For this review, take the finished solid that the model builds, in its own axes (mm). Face numbers are marked on the shaded views. A direction names the side the tool comes from. Coordinates: 2 decimals unless noted, no trailing zeros. Order: outer loops, then holes, each group sorted by start corner. A loop starts at its lowest first (then second) coordinate and runs counter-clockwise, first axis right, second up. Notation, with made-up numbers: M -18.5,86.5 L -5.5,86.5 A14 ccw -5.5,104.5 Z; hole C -18.75,46 d1. An arc over 180 degrees is marked long. Use one line per item in the form item = value. Start each with the question number.
```python
from build123d import *

# Parameters (mm, degrees)
HEX_CUT_DEPTH = 3.048
CHAMFER2_SIZE = 0.381


with BuildPart() as part:
    # Base Sketch → Base (revolve)
    with BuildSketch(Plane.XY, mode=Mode.PRIVATE) as base_sk:
        Polygon((0, 0), (25.4, 0), (25.4, 4.7625), (19.05, 4.7625), (19.05, 3.175), (0, 3.175), align=None)
    revolve(base_sk.sketch.rotate(Axis((0, 0, 0), (1, 0, 0)), 90), axis=Axis((0, 0, 0), (1, 0, 0)))

    # Hex Sketch → Hex Cut (cut)
    with BuildSketch(Plane(origin=(25.4, 0, 0), x_dir=(0, 0, -1), z_dir=(1, 0, 0))):
        Polygon((-1.374815329, 2.38125), (-2.749630657, 0), (-1.374815329, -2.38125), (1.374815329, -2.38125), (2.749630657, 0), (1.374815329, 2.38125), align=None)
    extrude(amount=-HEX_CUT_DEPTH, mode=Mode.SUBTRACT)

    # Chamfer2
    chamfer2_edges = [part.edges().sort_by_distance(p)[0] for p in [
        (0, 0, -3.175),
        (19.05, 0, -4.7625),
        (25.4, 0, -4.7625),
    ]]
    chamfer(chamfer2_edges, length=CHAMFER2_SIZE)


solid = part.part
```
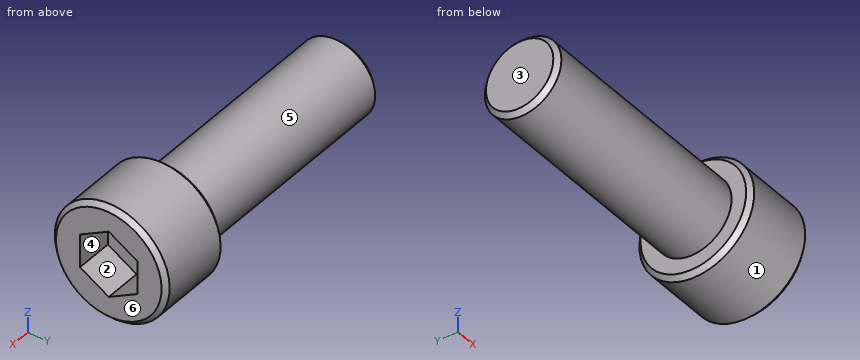
1. For pin 1 Ø5 at (x, y) = (19.5, 3) entering from -Z; pin 2 Ø2.5 at (y, z) = (-0.5, -0.5) entering from +X; pin 3 Ø2 at (x, z) = (4, 0) entering from +Y (3 decimals), all flat-tipped, find the tip position at first contact; note any pin that passes through.
2. Tool access review of the marked faces 5 and 6: name each direction out of +Z, -Z, +X, -X, +Y, -Y from which nothing blocks a thin tool from reaching the whole face with its end or side.
3. The part is to be moulded in two halves that separate along Z. For the marked faces 1, 2, 3 and 4, say which applies: pulls with the +Z half, pulls with the -Z half, needs draft (parallel to the pull), parting line crosses it, or undercut.
4. Consider section B-B, the plane x = 2. Write out the cut boundary in (y, z) (3 decimals), plus the area to 3 significant figures.
5. To check wall thickness, follow line 1 (Y direction, x = 1.25, z = 1.5); line 2 (X direction, y = 0.25, z = 2); line 3 (X direction, y = 1.75, z = 3.5). State the ranges of each line that lie inside material, in increasing order.
Answers follow:
q1.pin_1 = -4.74
q1.pin_2 = 22.35
q1.pin_3 = 3.175
q2.face_5 = -X
q2.face_6 = +Z, -Z, +X, +Y, -Y
q3.face_1 = parting line crosses it
q3.face_2 = undercut
q3.face_3 = needs draft
q3.face_4 = undercut
q4.outline = C 0,0 d6.35
q4.area = 31.7 mm²
q5.line_1 = -2.8 to 2.8
q5.line_2 = 0 to 22.35
q5.line_3 = 19.05 to 25.4
